Build history of the part. All positions in model axes, mm. A direction names the side the tool comes from. Round coordinates to 2 decimals unless told otherwise and drop trailing zeros. Order: outer loops, then holes, each group sorted by start corner. A loop starts at its lowest first (then second) coordinate and runs counter-clockwise, first axis right, second up. Notation, with made-up numbers: (74, 31) -> (133, 31) arc R27 cw to (133, 57) -> close; hole circle Ø4 at (-21, 16.5). An arc over 180 degrees is marked (long way). Answer as a JSON object with one key per item and string values.
from build123d import *

# Parameters (mm, degrees)
CUT_EXTRUDE1_REACH = 64.262
SKETCH5_R          = 5
CIRPATTERN1_COUNT  = 4


with BuildPart() as part:
    # Sketch4 → Revolve1 (revolve)
    with BuildSketch(Plane.XY, mode=Mode.PRIVATE) as revolve1_sk:
        Polygon((11.25, 0), (11.25, 12), (19, 12), (27.5, 42), (32.5, 42), (22.5, 0), align=None)
    revolve(revolve1_sk.sketch.rotate(Axis((0, 0, 0), (0, 1, 0)), 90), axis=Axis((0, 0, 0), (0, 1, 0)))

    # Cut-Extrude1: up to this cone (the profile starts inside it)
    cut_extrude1_end = Plane(origin=(0, 42, 0), z_dir=(0, 1, 0)) * Cone(9.342380952, 55.657619048, 194.524, mode=Mode.PRIVATE)
    # Sketch5 → Cut-Extrude1 (cut, up to the surface)
    with BuildSketch(Plane.XY, mode=Mode.PRIVATE) as cut_extrude1_sk1:
        with Locations((0, 42)):
            Circle(SKETCH5_R)
    cut_extrude1_tool1 = extrude(cut_extrude1_sk1.sketch, amount=-CUT_EXTRUDE1_REACH, mode=Mode.PRIVATE) & cut_extrude1_end
    cut_extrude1 = cut_extrude1_tool1.solids().sort_by_distance((0, 42, 0))[0]
    add(cut_extrude1, mode=Mode.SUBTRACT)

    # CirPattern1: Cut-Extrude1 ×4 about axis
    cirpattern1_axis = Axis((0, 42, 0), (0, -1, 0))
    for i in range(1, CIRPATTERN1_COUNT):
        add(cut_extrude1.rotate(cirpattern1_axis, i * 360 / CIRPATTERN1_COUNT), mode=Mode.SUBTRACT)


solid = part.part
1) Cut at C-C, the plane y = 28. Give the cut face in (x, z).
Checked values:
{"outline": "circle Ø58.33 at (0, 0); hole circle Ø47.07 at (0, 0)"}
2) Cut at A-A, the plane x = 0. Give the cut face in (y, z).
Checked values:
{"outline": "(0, -22.5) -> (37, -31.31) -> (37, -26.08) -> (12, -19) -> (12, -11.25) -> (0, -11.25) -> close; (0, 11.25) -> (12, 11.25) -> (12, 19) -> (37, 26.08) -> (37, 31.31) -> (0, 22.5) -> close"}
3) Flat gauge pins, fed straight in: pin 1 Ø12 at (x, z) = (22.5, 24.5) entering from +Y; pin 2 Ø10 at (x, y) = (19.5, 22) entering from -Z; pin 3 Ø8 at (x, y) = (-16, 26.5) entering from +Z; pin 4 Ø3 at (x, z) = (-11, -11) entering from +Y. Where does each tip first touch, or does it go through?
Checked values:
{"pin 1": "stops at y = 42", "pin 2": "stops at z = -23.95", "pin 3": "stops at z = 26.47", "pin 4": "stops at y = 12"}
4) Which spindle directions (+Z, -Z, +X, -X, +Y, -Y) get a long thin tool onto all of the face, cutting with end or side? Do faces 1 (the face through (8.2, 12, 8.2)), 2 (the face through (9.98, 6.08, -5.19)). Say none if no direction does.
Checked values:
{"face 1": "+Y", "face 2": "+Y, -Y"}
5) Cut at B-B, the plane y = 35. Give the cut face in (x, z).
Checked values:
{"outline": "circle Ø61.67 at (0, 0); hole circle Ø51.03 at (0, 0)"}
6) Probe L1, parallel to Z at x = 18, y = 20.5; L2, parallel to X at y = 2, z = 3; L3, parallel to Y at x = 10, z = 15.5. List the from-to ranges inside material, lowest first. Write a range as from..to.
Checked values:
{"L1": "z = -20.63..-11.59, 11.59..20.63", "L2": "x = -22.78..-10.84, 10.84..22.78", "L3": "y = 0..12"}
7) Pull direction Z, two halves, no side cores. Call faces 3 (the face through (0, 37, -29)), 4 (the face through (29, 37, 0)), 5 (the face through (23.35, 16.04, -12.14)): pulls with the +Z half, pulls with the -Z half, needs draft (parallel to the pull), parting line crosses it, or undercut.
Checked values:
{"face 3": "needs draft", "face 4": "undercut", "face 5": "parting line crosses it"}
